The listing builds one solid part. Answer for the finished solid, in the listing's coordinates (mm). Round coordinates to 2 decimals unless told otherwise and drop trailing zeros. Order: outer loops, then holes, each group sorted by start corner. A loop starts at its lowest first (then second) coordinate and runs counter-clockwise, first axis right, second up. Notation, with made-up numbers: M 6.25,11.5 L 22.25,11.5 A24 ccw 22.25,25.5 Z; hole C -8.75,24 d8. An arc over 180 degrees is marked long. Put each result on its own line as item: value. Start each with the question number.
1. The part is cut by section A-A (z = -6). Give the vertices of the cut face in (x, y).
2. Consider line 1 (X direction, y = 0.85, z = -28.05); line 2 (Z direction, x = 50.5, y = 0.55); line 3 (X direction, y = 0.5, z = -14). Determine where each line is inside the solid, lowest interval first.
3. The part is cut by section B-B (x = -1). Give the vertices of the cut face in (y, z), then the cut area to 3 significant figures.
4. This flat-tipped pin is pushed along its axis until it touches: pin 1 Ø0.8 at (y, z) = (1.5, -21.5) entering from -X. Where does it stop, or does it pass through?
5. The part is cut by section D-D (x = 44). Give the vertices of the cut face in (y, z).
6. The part is cut by section C-C (y = 1.6). Count the separate pieces of the cut face and the enclosed holes in it, then the cut area to 3 significant figures.
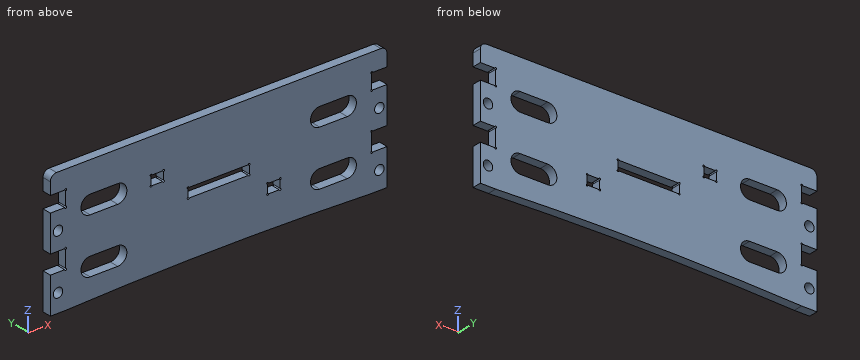
from build123d import *

# Parameters (mm, degrees)
BOSS_EXTRUDE1_DEPTH = 3
SKETCH2_W           = 4.1
SKETCH2_H           = 3.1
CUT_EXTRUDE1_DEPTH  = 10
BOSS_EXTRUDE2_DEPTH = 3
FILLET2_R           = 2
SKETCH5_R           = 1.55
SKETCH5_W           = 20
SKETCH5_H           = 3.1
CUT_EXTRUDE3_DEPTH  = 3
CUT_EXTRUDE2_DEPTH  = 10


with BuildPart() as part:
    # Sketch1 → Boss-Extrude1 (new body)
    with BuildSketch(Plane(origin=(0, 0, 0), x_dir=(1, 0, 0), z_dir=(0, 1, 0))):
        with BuildLine():
            Line((55, 34), (55, 22.1))
            Line((55, 22.1), (50, 22.1))
            Line((50, 22.1), (50, 16))
            Line((50, 16), (55, 16))
            Line((55, 16), (55, 4.1))
            Line((55, 4.1), (50, 4.1))
            Line((50, 4.1), (50, 0))
            Line((50, 0), (-50, 0))
            Line((-50, 0), (-50, 4.1))
            Line((-50, 4.1), (-55, 4.1))
            Line((-55, 4.1), (-55, 16))
            Line((-55, 16), (-50, 16))
            Line((-50, 16), (-50, 22.1))
            Line((-50, 22.1), (-55, 22.1))
            Line((-55, 22.1), (-55, 34))
            Line((-55, 34), (-50, 34))
            ThreePointArc((-50, 34), (0, 33), (50, 34))
            Line((50, 34), (55, 34))
        make_face()
        with BuildLine():
            Line((33, 9), (42, 9))
            ThreePointArc((42, 9), (45, 6), (42, 3))
            Line((42, 3), (33, 3))
            ThreePointArc((33, 3), (30, 6), (33, 9))
        make_face(mode=Mode.SUBTRACT)
        with BuildLine():
            Line((-33, 21), (-42, 21))
            ThreePointArc((-42, 21), (-45, 24), (-42, 27))
            Line((-42, 27), (-33, 27))
            ThreePointArc((-33, 27), (-30, 24), (-33, 21))
        make_face(mode=Mode.SUBTRACT)
        with BuildLine():
            Line((42, 27), (33, 27))
            ThreePointArc((33, 27), (30, 24), (33, 21))
            Line((33, 21), (42, 21))
            ThreePointArc((42, 21), (45, 24), (42, 27))
        make_face(mode=Mode.SUBTRACT)
        with BuildLine():
            Line((-42, 3), (-33, 3))
            ThreePointArc((-33, 3), (-30, 6), (-33, 9))
            Line((-33, 9), (-42, 9))
            ThreePointArc((-42, 9), (-45, 6), (-42, 3))
        make_face(mode=Mode.SUBTRACT)
    extrude(amount=BOSS_EXTRUDE1_DEPTH)

    # Sketch2 → Cut-Extrude1 (cut)
    with BuildSketch(Plane(origin=(0, 3, 0), x_dir=(1, 0, 0), z_dir=(0, 1, 0))):
        with Locations((-20.05, 5.85)):
            Rectangle(SKETCH2_W, SKETCH2_H)
        with Locations((18.05, 21.15)):
            Rectangle(SKETCH2_W, SKETCH2_H)
    extrude(amount=-CUT_EXTRUDE1_DEPTH, mode=Mode.SUBTRACT)

    # Sketch3 → Boss-Extrude2 (add)
    with BuildSketch(Plane(origin=(0, 3, 0), x_dir=(1, 0, 0), z_dir=(0, 1, 0))):
        Polygon((-50, 0), (-50, -1), (-55, -1), (-55, -7), (55, -7), (55, -1), (50, -1), (50, 0), align=None)
    extrude(amount=-BOSS_EXTRUDE2_DEPTH)

    # Fillet2
    fillet2_edges = [part.edges().sort_by_distance(p)[0] for p in [
        (55, 1.5, 7),
        (-55, 1.5, 7),
    ]]
    fillet(fillet2_edges, radius=FILLET2_R)

    # Sketch5 → Cut-Extrude3 (cut)
    with BuildSketch(Plane(origin=(0, 3, 0), x_dir=(1, 0, 0), z_dir=(0, 1, 0))):
        with Locations(Location((52.5, 28.05, 0), (0, 0, 270))):
            Circle(SKETCH5_R)
        with Locations(Location((52.5, 10.05, 0), (0, 0, 270))):
            Circle(SKETCH5_R)
        with Locations(Location((-52.5, 28.05, 0), (0, 0, 270))):
            Circle(SKETCH5_R)
        with Locations(Location((-52.5, 10.05, 0), (0, 0, 270))):
            Circle(SKETCH5_R)
        with Locations((0, 13.55)):
            Rectangle(SKETCH5_W, SKETCH5_H)
    extrude(amount=-CUT_EXTRUDE3_DEPTH, mode=Mode.SUBTRACT)

    # Sketch4 → Cut-Extrude2 (cut)
    with BuildSketch(Plane(origin=(0, 3, 0), x_dir=(1, 0, 0), z_dir=(0, 1, 0))):
        with BuildLine():
            ThreePointArc((-50, 3.8), (-49.787867966, 4.312132034), (-50.3, 4.1))
            Line((-50.3, 4.1), (-50, 4.1))
            Line((-50, 4.1), (-50, 3.8))
        make_face()
        with BuildLine():
            Line((-50, -0.7), (-50, -1))
            Line((-50, -1), (-50.3, -1))
            ThreePointArc((-50.3, -1), (-49.787867966, -1.212132034), (-50, -0.7))
        make_face()
        with BuildLine():
            ThreePointArc((-50, 21.8), (-49.787867966, 22.312132034), (-50.3, 22.1))
            Line((-50.3, 22.1), (-50, 22.1))
            Line((-50, 22.1), (-50, 21.8))
        make_face()
        with BuildLine():
            ThreePointArc((-50.3, 16), (-49.787867966, 15.787867966), (-50, 16.3))
            Line((-50, 16.3), (-50, 16))
            Line((-50, 16), (-50.3, 16))
        make_face()
        with BuildLine():
            Line((50.3, 16), (50, 16))
            Line((50, 16), (50, 16.3))
            ThreePointArc((50, 16.3), (49.787867966, 15.787867966), (50.3, 16))
        make_face()
        with BuildLine():
            Line((50, 21.8), (50, 22.1))
            Line((50, 22.1), (50.3, 22.1))
            ThreePointArc((50.3, 22.1), (49.787867966, 22.312132034), (50, 21.8))
        make_face()
        with BuildLine():
            Line((50.3, -1), (50, -1))
            Line((50, -1), (50, -0.7))
            ThreePointArc((50, -0.7), (49.787867966, -1.212132034), (50.3, -1))
        make_face()
        with BuildLine():
            Line((50, 3.8), (50, 4.1))
            Line((50, 4.1), (50.3, 4.1))
            ThreePointArc((50.3, 4.1), (49.787867966, 4.312132034), (50, 3.8))
        make_face()
        with BuildLine():
            ThreePointArc((-21.8, 7.4), (-22.312132034, 7.612132034), (-22.1, 7.1))
            Line((-22.1, 7.1), (-22.1, 7.4))
            Line((-22.1, 7.4), (-21.8, 7.4))
        make_face()
        with BuildLine():
            ThreePointArc((-18, 7.1), (-17.787867966, 7.612132034), (-18.3, 7.4))
            Line((-18.3, 7.4), (-18, 7.4))
            Line((-18, 7.4), (-18, 7.1))
        make_face()
        with BuildLine():
            ThreePointArc((-18.3, 4.3), (-17.787867966, 4.087867966), (-18, 4.6))
            Line((-18, 4.6), (-18, 4.3))
            Line((-18, 4.3), (-18.3, 4.3))
        make_face()
        with BuildLine():
            ThreePointArc((-22.1, 4.6), (-22.312132034, 4.087867966), (-21.8, 4.3))
            Line((-21.8, 4.3), (-22.1, 4.3))
            Line((-22.1, 4.3), (-22.1, 4.6))
        make_face()
        with BuildLine():
            ThreePointArc((16.3, 22.7), (15.787867966, 22.912132034), (16, 22.4))
            Line((16, 22.4), (16, 22.7))
            Line((16, 22.7), (16.3, 22.7))
        make_face()
        with BuildLine():
            ThreePointArc((20.1, 22.4), (20.312132034, 22.912132034), (19.8, 22.7))
            Line((19.8, 22.7), (20.1, 22.7))
            Line((20.1, 22.7), (20.1, 22.4))
        make_face()
        with BuildLine():
            ThreePointArc((19.8, 19.6), (20.312132034, 19.387867966), (20.1, 19.9))
            Line((20.1, 19.9), (20.1, 19.6))
            Line((20.1, 19.6), (19.8, 19.6))
        make_face()
        with BuildLine():
            ThreePointArc((16, 19.9), (15.787867966, 19.387867966), (16.3, 19.6))
            Line((16.3, 19.6), (16, 19.6))
            Line((16, 19.6), (16, 19.9))
        make_face()
        with BuildLine():
            ThreePointArc((-9.7, 15.1), (-10.212132034, 15.312132034), (-10, 14.8))
            Line((-10, 14.8), (-10, 15.1))
            Line((-10, 15.1), (-9.7, 15.1))
        make_face()
        with BuildLine():
            ThreePointArc((10, 14.8), (10.212132034, 15.312132034), (9.7, 15.1))
            Line((9.7, 15.1), (10, 15.1))
            Line((10, 15.1), (10, 14.8))
        make_face()
        with BuildLine():
            ThreePointArc((9.7, 12), (10.212132034, 11.787867966), (10, 12.3))
            Line((10, 12.3), (10, 12))
            Line((10, 12), (9.7, 12))
        make_face()
        with BuildLine():
            ThreePointArc((-10, 12.3), (-10.212132034, 11.787867966), (-9.7, 12))
            Line((-9.7, 12), (-10, 12))
            Line((-10, 12), (-10, 12.3))
        make_face()
    extrude(amount=-CUT_EXTRUDE2_DEPTH, mode=Mode.SUBTRACT)


solid = part.part
Resolved:
1. outline: M -55,0 L -45,0 L -45,3 L -55,3 Z; M -30,0 L -22.1,0 L -22.1,3 L -30,3 Z; M -18,0 L 30,0 L 30,3 L -18,3 Z; M 45,0 L 55,0 L 55,3 L 45,3 Z
2. line 1: -55 to -54.05, -50.95 to 50.95, 54.05 to 55
2. line 2: -34 to -22.1, -16 to -4.1, 1 to 7
2. line 3: -55 to -10, 10 to 55
3. outline: M 0,-33 L 3,-33 L 3,-15.1 L 0,-15.1 Z; M 0,-12 L 3,-12 L 3,7 L 0,7 Z
3. area: 111 mm2
4. pin 1: x = -50
5. outline: M 0,-33.77 L 3,-33.77 L 3,-26.24 L 0,-26.24 Z; M 0,-21.76 L 3,-21.76 L 3,-8.24 L 0,-8.24 Z; M 0,-3.76 L 3,-3.76 L 3,7 L 0,7 Z
6. separate pieces: 1
6. enclosed holes: 11
6. area: 3,880 mm2
